Design review of the part built by this model. Coordinates are the model's own, in mm. A direction names the side the tool comes from. Coordinates: 2 decimals unless noted, no trailing zeros. Loops run counter-clockwise (first coordinate to the right, second up) from the corner with the lowest first, then second, coordinate; pieces in that order, holes last.
Q1. Add section C-C on x = -4.5. Give the boundary of the cut face in (y, z), and give its area (3 significant figures).
Q2. Add section B-B on z = 0. Give the boundary of the cut face in (x, y).
Q3. Machinability: for faces 3 (the face through (-4, -1, 0)), 4 (the face through (1.617, 20.74, 0.67)), 5 (the face through (-5.5, 0, 0)), 6 (the face through (4, 43, 0)), 7 (the face through (5.5, 42, 0)), which of the approach directions +Z, -Z, +X, -X, +Y, -Y give a long, thin tool a straight path to every point of the face, cutting with its end or side? Answer none if there is none.
Q4. For P1, Ø3, axis at x = 2.5, y = 10.5, coming from the -Z side; P2, Ø1.5, axis at x = 3, z = 1.5, coming from the -Y side; P3, Ø5, axis at x = 1, y = 11.5, coming from the -Z side, all flat-tipped, find the tip position at first contact; note any pin that passes through.
Q5. Add section D-D on x = 0. Give the boundary of the cut face in (y, z).
Q6. Add section A-A on y = 42. Give the boundary of the cut face in (x, z).
Q7. Wall thickness on probe 1 along Y at (x, z) = (0, -0.25); probe 2 along Z at (x, y) = (-1, 42); probe 3 along Y at (x, z) = (-2.5, 0.5): over which ranges is each line inside the solid? List them lowest first.
Q8. Draft analysis for pull direction Y (two halves, no side actions). For faces 1 (the face through (5.5, 0, 0)), 2 (the face through (-4, 43, 0)), state which applies: released by +Y, released by -Y, zero draft, split by the parting line, or undercut.
```python
from build123d import *

# Parameters (mm, degrees)
ESQUISSE3_R        = 1
BOSS_EXTRU_1_DEPTH = 5.5
CHANFREIN1_SIZE    = 0.25


with BuildPart() as part:
    # Esquisse1 → Base-Révolution (revolve)
    with BuildSketch(Plane.XY):
        with BuildLine():
            Line((1.75, 39.563301414), (1.75, 2.436698586))
            ThreePointArc((1.75, 2.436698586), (2.855704445, -0.919212772), (0, -3))
            Line((0, -3), (0, 45))
            ThreePointArc((0, 45), (2.855704445, 42.919212772), (1.75, 39.563301414))
        make_face()
    revolve(axis=Axis((0, -3, 0), (0, 1, 0)))

    # Esquisse3 → Boss.-Extru.1 (add, symmetric)
    with BuildSketch(Plane(origin=(0, 0, 0), x_dir=(0, 0, -1), z_dir=(1, 0, 0))):
        Circle(ESQUISSE3_R)
        with Locations((0, 42)):
            Circle(ESQUISSE3_R)
    extrude(amount=BOSS_EXTRU_1_DEPTH, both=True)

    # Chanfrein1
    chanfrein1_edges = [part.edges().sort_by_distance(p)[0] for p in [
        (5.5, 42, 1),
        (-5.5, 42, 1),
        (5.5, 0, 1),
        (-5.5, 0, 1),
    ]]
    chamfer(chanfrein1_edges, length=CHANFREIN1_SIZE)


solid = part.part
```
Entries:
1. outline: circle Ø2 at (0, 0); circle Ø2 at (42, 0)
1. area: 6.28 mm2
2. outline: (-5.5, -0.75) - (-5.25, -1) - (-2.83, -1) arc R3 ccw to (2.83, -1) - (5.25, -1) - (5.5, -0.75) - (5.5, 0.75) - (5.25, 1) - (2.83, 1) arc R3 ccw to (1.75, 2.44) - (1.75, 39.56) arc R3 ccw to (2.83, 41) - (5.25, 41) - (5.5, 41.25) - (5.5, 42.75) - (5.25, 43) - (2.83, 43) arc R3 ccw to (-2.83, 43) - (-5.25, 43) - (-5.5, 42.75) - (-5.5, 41.25) - (-5.25, 41) - (-2.83, 41) arc R3 ccw to (-1.75, 39.56) - (-1.75, 2.44) arc R3 ccw to (-2.83, 1) - (-5.25, 1) - (-5.5, 0.75) - close
3. face 3: -X
3. face 4: none
3. face 5: +Z, -Z, -X, +Y, -Y
3. face 6: +X
3. face 7: +Z, -Z, +X, +Y, -Y
4. P1: stops at z = -1.44
4. P2: stops at y = -1.49
4. P3: stops at z = -1.75
5. outline: (2.44, -1.75) - (39.56, -1.75) arc R3 ccw (long way) to (39.56, 1.75) - (2.44, 1.75) arc R3 ccw (long way) to start
6. outline: (-5.5, -0.75) - (-5.25, -1) - (-2.83, -1) arc R3 ccw to (2.83, -1) - (5.25, -1) - (5.5, -0.75) - (5.5, 0.75) - (5.25, 1) - (2.83, 1) arc R3 ccw to (-2.83, 1) - (-5.25, 1) - (-5.5, 0.75) - close
7. probe 1: y = -2.99 to 44.99
7. probe 2: z = -2.83 to 2.83
7. probe 3: y = -1.58 to 1.58, 40.42 to 43.58
8. face 1: zero draft
8. face 2: undercut
